Input: part model. Units: mm. Frame: model coordinates. Face numbers are marked on the shaded views. A direction names the side the tool comes from. Give positions to 0.01 mm unless a question says otherwise; leave off trailing zeros. Loops run counter-clockwise (first coordinate to the right, second up) from the corner with the lowest first, then second, coordinate; pieces in that order, holes last. Notation, with made-up numbers: (67.5, 78.5) - (86.5, 78.5) arc R17 ccw to (86.5, 102.5) - close; hole circle Ø6 at (63, -15). An arc over 180 degrees is marked (long way). Answer as a JSON object with one key per item and string values. Group by question number.
(1) Material intervals for L1, parallel to Y at x = 4.6, z = 18.05; L2, parallel to X at y = 4, z = 17.05; L3, parallel to Z at x = 3.5, y = 1.5, sorted ascending.
(2) Mould query, pull axis X, two halves, no side actions, for the marked faces 1, 2 and 3. Classes: +X half, -X half, draft (parallel to the pull), parting line (faces both ways), or undercut.
(3) Section query B-B (z = 7.25). Return loops of the section in (x, y), plus the area to 3 significant figures.
(4) Pin query (flat end, axial travel): P1, Ø1.5, axis at y = 5.5, z = 6.5, coming from the -X side; P2, Ø12, axis at y = 15, z = 9.5, coming from the -X side; P3, Ø6, axis at y = 12, z = 6, coming from the +X side; P4, Ø1.5, axis at x = 3, z = 18.5, coming from the +Y side. Return the tip coordinate at first contact, or that it passes through.
(5) Access query for the marked faces 4, 5, 6, 7 and 8. Directions: +Z, -Z, +X, -X, +Y, -Y. A direction counts if a zero-diameter tool reaches every point of the face in a straight line with its end or side. Return the directions, or none.
(6) Section query C-C (z = 4). Return loops of the section in (x, y), plus the area to 3 significant figures.
(7) Section query A-A (y = 4). Return loops of the section in (x, z), plus the area to 3 significant figures.
(8) Section query D-D (x = -17.5). Return loops of the section in (y, z), plus the area to 3 significant figures.
```python
from build123d import *

# Parameters (mm, degrees)
SKETCH2_R           = 1.6
BOSS_EXTRUDE1_DEPTH = 20
FILLET1_R           = 3
CUT_EXTRUDE1_REACH  = 52.685
SKETCH3_W           = 6
SKETCH3_H           = 10


with BuildPart() as part:
    # Sketch2 → Boss-Extrude1 (new body)
    with BuildSketch(Plane.XY):
        Polygon((-45, 0), (0, 0), (8, 0), (8, 8), (2, 8), (2, 20), (-3, 20), (-18, 5), (-45, 5), align=None)
        with Locations((4.6, 4)):
            Circle(SKETCH2_R, mode=Mode.SUBTRACT)
        Polygon((-3, 5), (-13.757359313, 5), (-3, 15.757359313), align=None, mode=Mode.SUBTRACT)
    extrude(amount=BOSS_EXTRUDE1_DEPTH)

    # Fillet1
    fillet1_edges = [part.edges().sort_by_distance(p)[0] for p in [
        (8, 8, 10),
        (8, 0, 10),
    ]]
    fillet(fillet1_edges, radius=FILLET1_R)

    # Sketch3 → Cut-Extrude1 (cut, up to next)
    with BuildSketch(Plane(origin=(0, 8, 0), x_dir=(1, 0, 0), z_dir=(0, 1, 0)), mode=Mode.PRIVATE) as cut_extrude1_sk1:
        with Locations((5, -10)):
            Rectangle(SKETCH3_W, SKETCH3_H)
    cut_extrude1_tool1 = extrude(cut_extrude1_sk1.sketch, amount=-CUT_EXTRUDE1_REACH, mode=Mode.PRIVATE) & part.part
    add(cut_extrude1_tool1.solids().sort_by_distance((5, 8, 10))[0], mode=Mode.SUBTRACT)


solid = part.part
```
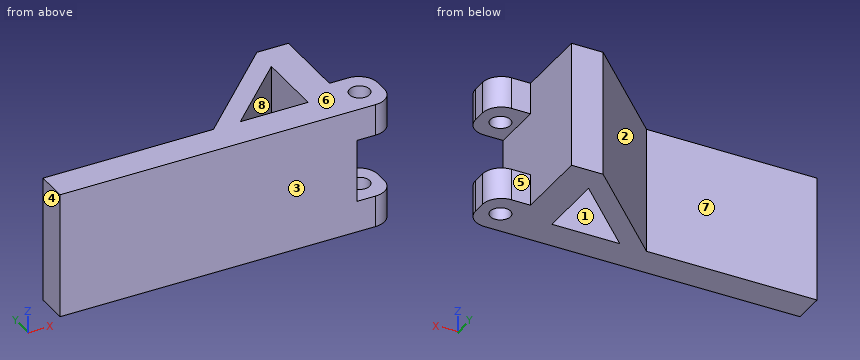
Recorded:
{
 "1": {"L1": "y = 0 to 2.4, 5.6 to 8", "L2": "x = -45 to 3, 6.2 to 8", "L3": "z = 0 to 5, 15 to 20"},
 "2": {"face 1": "undercut", "face 2": "-X half", "face 3": "draft"},
 "3": {"outline": "(-45, 0) - (2, 0) - (2, 20) - (-3, 20) - (-18, 5) - (-45, 5) - close; hole (-13.76, 5) - (-3, 5) - (-3, 15.76) - close", "area": "365 mm^2"},
 "4": {"P1": "stops at x = -45", "P2": "stops at x = -14", "P3": "stops at x = 2", "P4": "stops at y = 8"},
 "5": {"face 4": "+Z, -Z, -X, +Y, -Y", "face 5": "+Z, -Z, +X, +Y", "face 6": "+Z, +X, -X, +Y, -Y", "face 7": "+Z, -Z, -X, +Y", "face 8": "+Z, -Z"},
 "6": {"outline": "(-45, 0) - (5, 0) arc R3 ccw to (8, 3) - (8, 5) arc R3 ccw to (5, 8) - (2, 8) - (2, 20) - (-3, 20) - (-18, 5) - (-45, 5) - close; hole (-13.76, 5) - (-3, 5) - (-3, 15.76) - close; hole circle Ø3.2 at (4.6, 4)", "area": "401 mm^2"},
 "7": {"outline": "(-45, 0) - (3, 0) - (3, 5) - (2, 5) - (2, 15) - (3, 15) - (3, 20) - (-45, 20) - close; (6.2, 0) - (8, 0) - (8, 5) - (6.2, 5) - close; (6.2, 15) - (8, 15) - (8, 20) - (6.2, 20) - close", "area": "968 mm^2"},
 "8": {"outline": "(0, 0) - (5.5, 0) - (5.5, 20) - (0, 20) - close", "area": "110 mm^2"}
}
